```python
from build123d import *

# Parameters (mm, degrees)
SKETCH2_R          = 1.75
CUT_EXTRUDE1_DEPTH = 10


with BuildPart() as part:
    # Sketch1 → Revolve1 (revolve)
    with BuildSketch(Plane.XY, mode=Mode.PRIVATE) as revolve1_sk:
        Polygon((-5, 15), (-5, 3.5), (-11, 3.5), (-11, 0), (-3, 0), (-3, 15), align=None)
    revolve(revolve1_sk.sketch.rotate(Axis((0, 0, 0), (0, 1, 0)), 270), axis=Axis((0, 0, 0), (0, 1, 0)))

    # Sketch2 → Cut-Extrude1 (cut)
    with BuildSketch(Plane(origin=(0, 3.5, 0), x_dir=(1, 0, 0), z_dir=(0, 1, 0))):
        with Locations(Location((0, 8, 0), (0, 0, 270))):
            Circle(SKETCH2_R)
        with Locations(Location((8, 0, 0), (0, 0, 270))):
            Circle(SKETCH2_R)
        with Locations(Location((0, -8, 0), (0, 0, 270))):
            Circle(SKETCH2_R)
        with Locations(Location((-8, 0, 0), (0, 0, 270))):
            Circle(SKETCH2_R)
    extrude(amount=-CUT_EXTRUDE1_DEPTH, mode=Mode.SUBTRACT)


solid = part.part
```
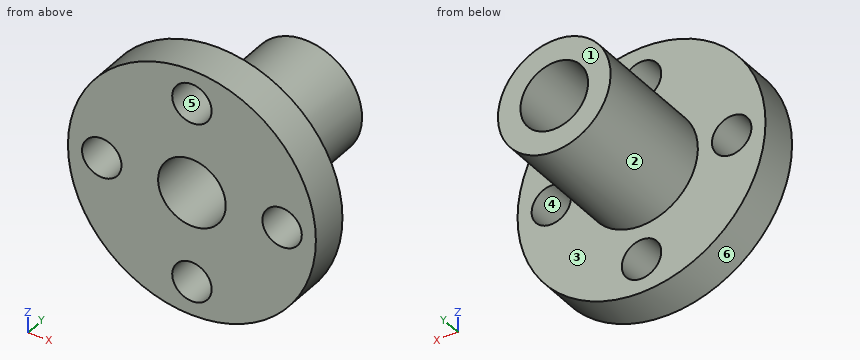
Geometry check sheet. Reference: the model listing, model coordinates, mm. Face numbers are marked on the shaded views. A direction names the side the tool comes from. Coordinates: 2 decimals unless noted, no trailing zeros. Order: outer loops, then holes, each group sorted by start corner. A loop starts at its lowest first (then second) coordinate and runs counter-clockwise, first axis right, second up. Notation, with made-up numbers: (-20.5, 19) - (1.5, 19) arc R32 cw to (1.5, 54) - close; hole circle Ø5 at (-18, 11.5). An arc over 180 degrees is marked (long way). Use one line per item in the form item = value.
1. Section check C-C (z = -8). Record the boundary of the cut face in (x, y), then the cut area to 3 significant figures.
Here are the results:
outline = (-7.55, 0) - (-1.75, 0) - (-1.75, 3.5) - (-7.55, 3.5) - close; (1.75, 0) - (7.55, 0) - (7.55, 3.5) - (1.75, 3.5) - close
area = 40.6 mm²
2. Access from +Z, -Z, +X, -X, +Y, -Y to the whole of each face (thin tool, end or side, straight path). Record for the marked faces 1 and 2.
Here are the results:
face_1 = +Z, -Z, +X, -X, +Y
face_2 = +Y
3. Scan lines: line 1 (X direction, y = 2.35, z = 0); line 2 (Y direction, x = 6.25, z = 8); line 3 (X direction, y = 1.05, z = 8). Record each from-to range of solid material in increasing order.
Here are the results:
line_1 = -11 to -9.75, -6.25 to -3, 3 to 6.25, 9.75 to 11
line_2 = 0 to 3.5
line_3 = -7.55 to -1.75, 1.75 to 7.55
4. Section check B-B (x = 8). Record the boundary of the cut face in (y, z).
Here are the results:
outline = (0, -7.55) - (3.5, -7.55) - (3.5, -1.75) - (0, -1.75) - close; (0, 1.75) - (3.5, 1.75) - (3.5, 7.55) - (0, 7.55) - close
5. Gauge pin test, flat ends, axial feed: pin 1 (5 mm diameter, centred on y = 7, z = -3, fed in from +X); pin 2 (1 mm diameter, centred on x = -5, y = 9.5, fed in from -Z); pin 3 (5 mm diameter, centred on x = -1.5, y = 7.5, fed in from -Z). Record the tip position at first contact, or that the pin passes through.
Here are the results:
pin_1 = 4.97
pin_2 = -2.18
pin_3 = -5
6. Section check D-D (y = 10.5). Record the boundary of the cut face in (x, z).
Here are the results:
outline = circle Ø10 at (0, 0); hole circle Ø6 at (0, 0)
7. Draft check along X on the marked faces 3, 4, 5 and 6. Enter one of: pulls with the +X half, pulls with the -X half, needs draft (parallel to the pull), parting line crosses it, or undercut.
Here are the results:
face_3 = needs draft
face_4 = undercut
face_5 = undercut
face_6 = parting line crosses it
8. Section check A-A (x = 0). Record the boundary of the cut face in (y, z).
Here are the results:
outline = (0, -11) - (3.5, -11) - (3.5, -9.75) - (0, -9.75) - close; (0, -6.25) - (3.5, -6.25) - (3.5, -5) - (15, -5) - (15, -3) - (0, -3) - close; (0, 3) - (15, 3) - (15, 5) - (3.5, 5) - (3.5, 6.25) - (0, 6.25) - close; (0, 9.75) - (3.5, 9.75) - (3.5, 11) - (0, 11) - close
